```python
from build123d import *

# Parameters (mm, degrees)
F1_DEPTH      = 2.5
F2_R          = 6.025
F3_DEPTH      = 25
F3_DEPTH_BACK = 25
F4_SIZE       = 0.2


with BuildPart() as f1:
    # F0 (on Front) → F1 (new body, symmetric)
    with BuildSketch(Plane.XZ):
        with BuildLine():
            Line((-64.5, 47.5), (-64.5, -37))
            ThreePointArc((-64.5, -37), (-41.5000010456, -60), (-18.5, -37.0000020911))
            Line((-18.5, -37.0000020911), (-21.9976072653, 29.7383202188))
            ThreePointArc((-21.9976072653, 29.7383202188), (-20.6313314466, 33.4417728785), (-17.0044595916, 35))
            Line((-17.0044595916, 35), (52, 35))
            ThreePointArc((52, 35), (64.5, 47.5), (52, 60))
            Line((52, 60), (-52, 60))
            ThreePointArc((-52, 60), (-60.8388347648, 56.3388347648), (-64.5, 47.5))
        make_face()
    extrude(amount=F1_DEPTH, both=True)

    # F2 (on Front) → F3 (cut, two sides)
    with BuildSketch(Plane.XZ) as f3_sk:
        with Locations((-41.5, -37)):
            Circle(F2_R)
        with Locations((-52, 47.5)):
            Circle(F2_R)
        with Locations((49.5, 47.5)):
            Circle(F2_R)
    extrude(amount=-F3_DEPTH, mode=Mode.SUBTRACT)
    extrude(f3_sk.sketch, amount=F3_DEPTH_BACK, mode=Mode.SUBTRACT)

    # F4
    f4_edges = [f1.edges().sort_by_distance(p)[0] for p in [
        (-20.631331, -2.5, 33.441773),
        (-20.248804, -2.5, -3.630841),
        (17.49777, -2.5, 35),
        (-41.500001, -2.5, -60),
        (64.5, -2.5, 47.5),
        (-64.5, -2.5, 5.25),
        (0, -2.5, 60),
        (-60.838835, -2.5, 56.338835),
        (-47.525, -2.5, -37),
        (-58.025, -2.5, 47.5),
        (43.475, -2.5, 47.5),
        (-20.631331, 2.5, 33.441773),
        (-20.248804, 2.5, -3.630841),
        (17.49777, 2.5, 35),
        (-41.500001, 2.5, -60),
        (64.5, 2.5, 47.5),
        (-64.5, 2.5, 5.25),
        (0, 2.5, 60),
        (-60.838835, 2.5, 56.338835),
        (-47.525, 2.5, -37),
        (-58.025, 2.5, 47.5),
        (43.475, 2.5, 47.5),
    ]]
    chamfer(f4_edges, length=F4_SIZE)


solid = f1.part
```
Geometry check sheet. Reference: the model listing, model coordinates, mm. Round coordinates to 2 decimals unless told otherwise and drop trailing zeros. Order: outer loops, then holes, each group sorted by start corner. A loop starts at its lowest first (then second) coordinate and runs counter-clockwise, first axis right, second up. Notation, with made-up numbers: M 46,53.5 L 103,53.5 A4 ccw 103,59.5 Z; hole C 47.5,10.5 d5. An arc over 180 degrees is marked long. Write item = value, one per line.
Q1. Section check C-C (z = -10.5). Enter the section's corners in (x, y).
Answer block:
outline = M -64.5,-2.3 L -64.3,-2.5 L -20.09,-2.5 L -19.89,-2.3 L -19.89,2.3 L -20.09,2.5 L -64.3,2.5 L -64.5,2.3 Z
Q2. Section check B-B (x = -41.5). Enter the section's corners in (y, z) (3 decimals).
Answer block:
outline = M -2.5,-59.8 L -2.3,-60 L 2.3,-60 L 2.5,-59.8 L 2.5,-43.225 L 2.3,-43.025 L -2.3,-43.025 L -2.5,-43.225 Z; M -2.5,-30.775 L -2.3,-30.975 L 2.3,-30.975 L 2.5,-30.775 L 2.5,59.8 L 2.3,60 L -2.3,60 L -2.5,59.8 Z
Q3. Depth check by flat-ended pin: pin 1 Ø9.5 at (x, z) = (-52, 47.5) entering from +Y. Enter the tip coordinate at first touch or a pass-through.
Answer block:
pin_1 = through
Q4. Scan lines: line 1 (X direction, y = -0.8, z = -37) (3 decimals); line 2 (X direction, y = 0.2, z = 47.5) (3 decimals); line 3 (Z direction, x = 49.5, y = 0.5) (3 decimals). Record each from-to range of solid material in increasing order.
Answer block:
line_1 = -64.5 to -47.525, -35.475 to -18.5
line_2 = -64.5 to -58.025, -45.975 to 43.475, 55.525 to 64.5
line_3 = 35 to 41.475, 53.525 to 60
Q5. Section check D-D (z = 2). Enter the section's corners in (x, y), plus the area to 3 significant figures.
Answer block:
outline = M -64.5,-2.3 L -64.3,-2.5 L -20.74,-2.5 L -20.54,-2.3 L -20.54,2.3 L -20.74,2.5 L -64.3,2.5 L -64.5,2.3 Z
area = 220 mm^2
Q6. Section check A-A (y = 0.65). Enter the section's corners in (x, z) (3 decimals), plus the area to 3 significant figures.
Answer block:
outline = M -64.5,-37 A23 ccw -18.5,-37 L -21.998,29.738 A5 cw -17.004,35 L 52,35 A12.5 ccw 52,60 L -52,60 A12.5 ccw -64.5,47.5 Z; hole C -52,47.5 d12.05; hole C -41.5,-37 d12.05; hole C 49.5,47.5 d12.05
area = 6,800 mm^2
Q7. Release check for a two-part mould opening along X. For faces 1 (the cylindrical face through (-60.741, -0.032, 56.435)), 2 (the cylindrical face through (52.74, -0.03, 52.58)), 3 (the cylindrical face through (64.497, -0.032, 47.225)) record: released by +X, released by -X, zero draft, split by the parting line, or undercut.
Answer block:
face_1 = released by -X
face_2 = undercut
face_3 = released by +X
